Read the model definition and answer for the solid it produces. Units are mm, in the model's axes. Face numbers are marked on the shaded views. A direction names the side the tool comes from. Coordinates: 2 decimals unless noted, no trailing zeros. Order: outer loops, then holes, each group sorted by start corner. A loop starts at its lowest first (then second) coordinate and runs counter-clockwise, first axis right, second up. Notation, with made-up numbers: (-16, 37) -> (41, 37) arc R11 ccw to (41, 54) -> close; hole circle Ø11 at (14.5, 40.25). An arc over 180 degrees is marked (long way). Answer as a JSON object with one key per item and string values. Group by question number.
1) Consider L1, parallel to X at y = 20, z = -69. Determine where the line is inside the solid, lowest interval first.
2) A tool of negligible diameter and unlimited length cuts with its end or side. For the marked faces 1 and 2, from which of +Z, -Z, +X, -X, +Y, -Y can it reach the whole face along a straight path? Write none if from no direction.
3) Section C-C on x = 14 is taken. Determine the outline of the cut face in (y, z), and give its area (3 significant figures).
4) Given pin 1 (3 mm diameter, centred on x = 9.5, y = 18, fed in from -Z); pin 2 (4 mm diameter, centred on x = 3, z = -14, fed in from +Y), each flat-ended and moving along its own axis, determine where each tip first touches the part or whether it passes through.
5) Section B-B on z = -23.5 is taken. Determine the outline of the cut face in (x, y), and give its area (3 significant figures).
6) Section A-A on y = -1 is taken. Determine the outline of the cut face in (x, z), and give its area (3 significant figures).
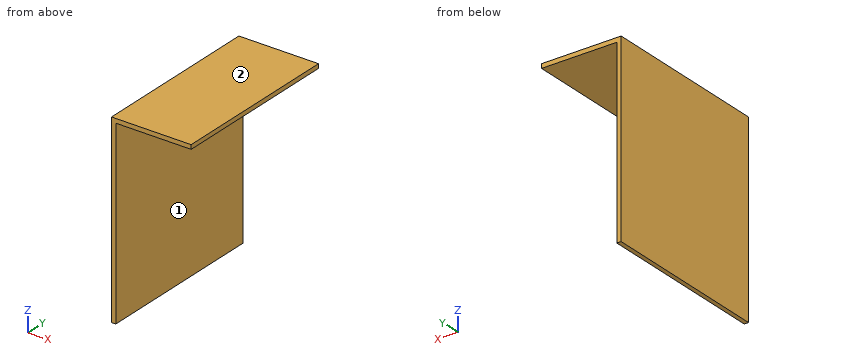
from build123d import *

# Parameters (mm, degrees)
SKETCH_1_W      = 2
SKETCH_1_H      = 87
EXTRUDE_1_DEPTH = 40
SKETCH_2_W      = 2
SKETCH_2_H      = 80
EXTRUDE_2_DEPTH = 35


with BuildPart() as part:
    # 草图1 → 凸台-拉伸1 (new body, symmetric)
    with BuildSketch(Plane(origin=(0, 0, 0), x_dir=(1, 0, 0), z_dir=(0, 1, 0))):
        with Locations((-1, 43.5)):
            Rectangle(SKETCH_1_W, SKETCH_1_H)
    extrude(amount=EXTRUDE_1_DEPTH, both=True)

    # 草图2 → 凸台-拉伸2 (add)
    with BuildSketch(Plane(origin=(0, 0, 0), x_dir=(0, 0, -1), z_dir=(1, 0, 0))):
        with Locations((1, 0)):
            Rectangle(SKETCH_2_W, SKETCH_2_H)
    extrude(amount=EXTRUDE_2_DEPTH)


solid = part.part
Worked answers:
{
 "1": {"L1": "x = -2 to 0"},
 "2": {"face 1": "-Z, +X, +Y, -Y", "face 2": "+Z, +X, -X, +Y, -Y"},
 "3": {"outline": "(-40, -2) -> (40, -2) -> (40, 0) -> (-40, 0) -> close", "area": "160 mm²"},
 "4": {"pin 1": "stops at z = -2", "pin 2": "passes through"},
 "5": {"outline": "(-2, -40) -> (0, -40) -> (0, 40) -> (-2, 40) -> close", "area": "160 mm²"},
 "6": {"outline": "(-2, -87) -> (0, -87) -> (0, -2) -> (35, -2) -> (35, 0) -> (-2, 0) -> close", "area": "244 mm²"}
}
